from build123d import *

# Parameters (mm, degrees)
F1_DEPTH = 63.5
F2_W     = 12.7
F2_H     = 7.62
F3_DEPTH = 25.4


with BuildPart() as f1:
    # F0 (on Right) → F1 (new body)
    with BuildSketch(Plane.YZ):
        Polygon((0, 71.12), (0, 0), (147.32, 0), (20.32, 71.12), align=None)
    extrude(amount=F1_DEPTH)

    # F2 (on Front) → F3 (cut)
    with BuildSketch(Plane.XZ):
        with Locations((31.75, 3.81)):
            Rectangle(F2_W, F2_H)
    extrude(amount=-F3_DEPTH, mode=Mode.SUBTRACT)


solid = f1.part
Work out the finished part from the listing and answer in its coordinate system (mm). A direction names the side the tool comes from. Give positions to 0.01 mm unless a question says otherwise; leave off trailing zeros. Order: outer loops, then holes, each group sorted by start corner. A loop starts at its lowest first (then second) coordinate and runs counter-clockwise, first axis right, second up. Notation, with made-up numbers: (72, 31) -> (77, 31) arc R20 cw to (77, 47) -> close; hole circle Ø6 at (-33.5, 24.25). An arc over 180 degrees is marked (long way). Answer as a JSON object with one key per item and string values. Group by question number.
1. Section B-B on x = 12 is taken. Determine the outline of the cut face in (y, z).
2. Section C-C on z = 63 is taken. Determine the outline of the cut face in (x, y).
3. Section A-A on y = 10.5 is taken. Determine the outline of the cut face in (x, z), plus the area to 3 significant figures.
4. Flat-ended cylindrical pins translate along their axes: pin 1 Ø4 at (x, y) = (32, 10) entering from -Z; pin 2 Ø2.5 at (x, z) = (32.5, 3) entering from -Y; pin 3 Ø1 at (x, z) = (12, 62) entering from +Y. Find the tip coordinate at first contact, or state that the pin passes through.
5. The mould has two halves that part along X. Classify faces 3 (the flat face through (32, 25.4, 4)), 4 (the flat face through (31, 10, 71.12)), 5 (the flat face through (0, 56, 28)), 6 (the flat face through (38.1, 13, 4)): released by +X, released by -X, zero draft, split by the parting line, or undercut.
6. Consider line 1 along Z through (x, y) = (36.5, 16); line 2 along Y through (x, z) = (34.5, 68.5); line 3 along Z through (x, y) = (30, 103). Determine where each line is inside the solid, lowest interval first. Write a range as [from, to].
7. Section D-D on x = 29.5 is taken. Determine the outline of the cut face in (y, z), plus the area to 3 significant figures.
8. A tool of negligible diameter and unlimited length cuts with its end or side. For faces 1 (the flat face through (25.4, 13, 4)), 2 (the flat face through (63.5, 56, 28)), from which of +Z, -Z, +X, -X, +Y, -Y can it reach the whole face along a straight path? Write none if from no direction.
Result sheet:
{
 "1": {"outline": "(0, 0) -> (147.32, 0) -> (20.32, 71.12) -> (0, 71.12) -> close"},
 "2": {"outline": "(0, 0) -> (63.5, 0) -> (63.5, 34.82) -> (0, 34.82) -> close"},
 "3": {"outline": "(0, 0) -> (25.4, 0) -> (25.4, 7.62) -> (38.1, 7.62) -> (38.1, 0) -> (63.5, 0) -> (63.5, 71.12) -> (0, 71.12) -> close", "area": "4,420 mm^2"},
 "4": {"pin 1": "stops at z = 7.62", "pin 2": "stops at y = 25.4", "pin 3": "stops at y = 37.5"},
 "5": {"face 3": "undercut", "face 4": "zero draft", "face 5": "released by -X", "face 6": "undercut"},
 "6": {"line 1": "z = [7.62, 71.12]", "line 2": "y = [0, 25]", "line 3": "z = [0, 24.82]"},
 "7": {"outline": "(0, 7.62) -> (25.4, 7.62) -> (25.4, 0) -> (147.32, 0) -> (20.32, 71.12) -> (0, 71.12) -> close", "area": "5,770 mm^2"},
 "8": {"face 1": "-Z, -Y", "face 2": "+Z, -Z, +X, +Y, -Y"}
}
